Part model, mm, in its own coordinate system. A direction names the side the tool comes from. Round coordinates to 2 decimals unless told otherwise and drop trailing zeros. Loops run counter-clockwise (first coordinate to the right, second up) from the corner with the lowest first, then second, coordinate; pieces in that order, holes last. Notation, with made-up numbers: (-28, 74) - (29, 74) arc R10 cw to (29, 80) - close; hole circle Ø8 at (0.25, 88.25). An arc over 180 degrees is marked (long way). Write each question's results on one line, items separated by ' | '. Start each with the question number.
(1) Drill centre lines: L1, parallel to X at y = 0, z = -8.5; L2, parallel to Y at x = 0, z = -5; L3, parallel to X at y = 0.5, z = -3. Where is each one in solid material? Low to high.
(2) Flat gauge pins, fed straight in: P1, Ø1, axis at x = -1, y = -0.5, coming from the -Z side; P2, Ø1, axis at y = 3.5, z = -1.5, coming from the +X side; P3, Ø1.5, axis at y = 2, z = -1, coming from the -X side. Where does each tip first touch, or does it go through?
(3) Cut at A-A, the plane z = 3.75. List the corners of the cut face in (x, y), then the cut area to 3 significant figures.
(4) Cut at D-D, the plane y = 0. List the corners of the cut face in (x, z).
(5) Cut at C-C, the plane z = -7.75. List the corners of the cut face in (x, y).
(6) Mould opens along X. For faces 6 (the face through (-6.2, 0, 0)), 7 (the face through (-5.95, 0.78, -4.93)), 8 (the face through (0, -2, -6)) say: released by +X, released by -X, zero draft, split by the parting line, or undercut.
(7) Cut at B-B, the plane y = -3.75. List the corners of the cut face in (x, z).
(8) Tool access for faces 1 (the face through (3.2, -5.4, 0)), 2 (the face through (-3, 5.4, 0)), 3 (the face through (-3, -5.4, 0)), 4 (the face through (3.2, 5.4, 0)), 5 (the face through (0, 1.476, -6)): list every direction of +Z, -Z, +X, -X, +Y, -Y with a clear straight run to the whole face (end or side of a thin tool).
from build123d import *

# Parameters (mm, degrees)
BOSS_EXTRUDE1_DEPTH = 8
SKETCH2_R           = 6
BOSS_EXTRUDE2_DEPTH = 10
CUT_EXTRUDE1_DEPTH  = 8
FILLET1_R           = 0.5


with BuildPart() as part:
    # Sketch1 → Boss-Extrude1 (new body)
    with BuildSketch(Plane.XY):
        Polygon((-3.464101615, -6), (3.464101615, -6), (6.92820323, 0), (3.464101615, 6), (-3.464101615, 6), (-6.92820323, 0), align=None)
    extrude(amount=BOSS_EXTRUDE1_DEPTH)

    # Sketch2 → Boss-Extrude2 (add)
    with BuildSketch(Plane(origin=(0, 0, 0), x_dir=(-1, 0, 0), z_dir=(0, 0, -1))):
        with Locations(Location((0, 0, 0), (0, 0, 150))):
            Circle(SKETCH2_R)
    extrude(amount=BOSS_EXTRUDE2_DEPTH)

    # Sketch3 → Cut-Extrude1 (cut)
    with BuildSketch(Plane(origin=(0, 0, -10), x_dir=(-1, 0, 0), z_dir=(0, 0, -1))):
        with BuildLine():
            Line((-1.35, 1.475635456), (1.35, 1.475635456))
            ThreePointArc((1.35, 1.475635456), (0, -2), (-1.35, 1.475635456))
        make_face()
    extrude(amount=-CUT_EXTRUDE1_DEPTH, mode=Mode.SUBTRACT)

    # Fillet1
    fillet1_edges = [part.edges().sort_by_distance(p)[0] for p in [
        (3.464101615, -6, 4),
        (-3.464101615, -6, 4),
        (-6.92820323, 0, 4),
        (-3.464101615, 6, 4),
        (3.464101615, 6, 4),
        (6.92820323, 0, 4),
    ]]
    fillet(fillet1_edges, radius=FILLET1_R)


solid = part.part
A:
1) L1: -6 to -2, 2 to 6 | L2: -6 to -2, 1.48 to 6 | L3: -5.98 to -1.94, 1.94 to 5.98
2) P1: z = -2 | P2: x = 5.2 | P3: x = -5.87
3) outline: (-6.78, -0.25) - (-3.61, -5.75) arc R0.5 ccw to (-3.18, -6) - (3.18, -6) arc R0.5 ccw to (3.61, -5.75) - (6.78, -0.25) arc R0.5 ccw to (6.78, 0.25) - (3.61, 5.75) arc R0.5 ccw to (3.18, 6) - (-3.18, 6) arc R0.5 ccw to (-3.61, 5.75) - (-6.78, 0.25) arc R0.5 ccw to start | area: 125 mm2
4) outline: (-6.85, 0) - (-6, 0) - (-6, -10) - (-2, -10) - (-2, -2) - (2, -2) - (2, -10) - (6, -10) - (6, 0) - (6.85, 0) - (6.85, 8) - (-6.85, 8) - close
5) outline: circle Ø12 at (0, 0); hole (-1.35, 1.48) arc R2 ccw (long way) to (1.35, 1.48) - close
6) face 6: zero draft | face 7: split by the parting line | face 8: undercut
7) outline: (-4.76, 0) - (-4.68, 0) - (-4.68, -10) - (4.68, -10) - (4.68, 0) - (4.76, 0) - (4.76, 8) - (-4.76, 8) - close
8) face 1: -Z, +X, -Y | face 2: -Z, -X, +Y | face 3: -Z, -X, -Y | face 4: -Z, +X, +Y | face 5: -Z
